from build123d import *

# Parameters (mm, degrees)
SKETCH1_W           = 25
SKETCH1_H           = 23.86
BOSS_EXTRUDE1_DEPTH = 1.12
SKETCH4_W           = 10.8
SKETCH4_H           = 10.8
BOSS_EXTRUDE2_DEPTH = 3.875
SKETCH5_R           = 2.375
CUT_EXTRUDE1_DEPTH  = 0.7
CUT_EXTRUDE2_REACH  = 19.708
SKETCH6_R           = 1.1
SKETCH8_R           = 1
BOSS_EXTRUDE3_DEPTH = 6.98
SKETCH9_W           = 25
SKETCH9_H           = 5.71
BOSS_EXTRUDE4_DEPTH = 2.75
FILLET1_R           = 1.5


with BuildPart() as part:
    # Sketch1 → Boss-Extrude1 (new body)
    with BuildSketch(Plane.XY):
        Rectangle(SKETCH1_W, SKETCH1_H)
    extrude(amount=BOSS_EXTRUDE1_DEPTH)

    # Sketch4 → Boss-Extrude2 (add)
    with BuildSketch(Plane.XY.offset(1.12)):
        with Locations((0, 2.2016)):
            Rectangle(SKETCH4_W, SKETCH4_H)
    extrude(amount=BOSS_EXTRUDE2_DEPTH)

    # Sketch5 → Cut-Extrude1 (cut)
    with BuildSketch(Plane.XY.offset(1.12)):
        with Locations((11, 2.2016)):
            Circle(SKETCH5_R)
        with Locations((11, -10.4984)):
            Circle(SKETCH5_R)
        with Locations((-11, -10.4984)):
            Circle(SKETCH5_R)
        with Locations((-11, 2.2016)):
            Circle(SKETCH5_R)
    extrude(amount=-CUT_EXTRUDE1_DEPTH, mode=Mode.SUBTRACT)

    # Sketch6 → Cut-Extrude2 (cut, up to next)
    with BuildSketch(Plane.XY.offset(1.12), mode=Mode.PRIVATE) as cut_extrude2_sk1:
        with Locations((11, 2.2016)):
            Circle(SKETCH6_R)
    cut_extrude2_tool1 = extrude(cut_extrude2_sk1.sketch, amount=-CUT_EXTRUDE2_REACH, mode=Mode.PRIVATE) & part.part
    # Sketch6 → Cut-Extrude2 (cut, up to next)
    with BuildSketch(Plane.XY.offset(1.12), mode=Mode.PRIVATE) as cut_extrude2_sk2:
        with Locations((11, -10.4984)):
            Circle(SKETCH6_R)
    cut_extrude2_tool2 = extrude(cut_extrude2_sk2.sketch, amount=-CUT_EXTRUDE2_REACH, mode=Mode.PRIVATE) & part.part
    # Sketch6 → Cut-Extrude2 (cut, up to next)
    with BuildSketch(Plane.XY.offset(1.12), mode=Mode.PRIVATE) as cut_extrude2_sk3:
        with Locations((-11, -10.4984)):
            Circle(SKETCH6_R)
    cut_extrude2_tool3 = extrude(cut_extrude2_sk3.sketch, amount=-CUT_EXTRUDE2_REACH, mode=Mode.PRIVATE) & part.part
    # Sketch6 → Cut-Extrude2 (cut, up to next)
    with BuildSketch(Plane.XY.offset(1.12), mode=Mode.PRIVATE) as cut_extrude2_sk4:
        with Locations((-11, 2.2016)):
            Circle(SKETCH6_R)
    cut_extrude2_tool4 = extrude(cut_extrude2_sk4.sketch, amount=-CUT_EXTRUDE2_REACH, mode=Mode.PRIVATE) & part.part
    add(cut_extrude2_tool1.solids().sort_by_distance((11, 2.2016, 1.12))[0], mode=Mode.SUBTRACT)
    add(cut_extrude2_tool2.solids().sort_by_distance((11, -10.4984, 1.12))[0], mode=Mode.SUBTRACT)
    add(cut_extrude2_tool3.solids().sort_by_distance((-11, -10.4984, 1.12))[0], mode=Mode.SUBTRACT)
    add(cut_extrude2_tool4.solids().sort_by_distance((-11, 2.2016, 1.12))[0], mode=Mode.SUBTRACT)

    # Sketch8 → Boss-Extrude3 (add)
    with BuildSketch(Plane.XY.offset(1.12)):
        with BuildLine():
            Line((2.875, 4.0766), (2.875, 0.3266))
            ThreePointArc((2.875, 0.3266), (2.582106781, -0.380506781), (1.875, -0.6734))
            Line((1.875, -0.6734), (-1.875, -0.6734))
            ThreePointArc((-1.875, -0.6734), (-2.582106781, -0.380506781), (-2.875, 0.3266))
            Line((-2.875, 0.3266), (-2.875, 4.0766))
            ThreePointArc((-2.875, 4.0766), (-2.582106781, 4.783706781), (-1.875, 5.0766))
            Line((-1.875, 5.0766), (1.875, 5.0766))
            ThreePointArc((1.875, 5.0766), (2.582106781, 4.783706781), (2.875, 4.0766))
        make_face()
        with Locations((0, 2.2016)):
            Circle(SKETCH8_R, mode=Mode.SUBTRACT)
    extrude(amount=BOSS_EXTRUDE3_DEPTH)

    # Sketch9 → Boss-Extrude4 (add)
    with BuildSketch(Plane(origin=(0, 0, 0), x_dir=(-1, 0, 0), z_dir=(0, 0, -1))):
        with Locations((0, 9.075)):
            Rectangle(SKETCH9_W, SKETCH9_H)
    extrude(amount=BOSS_EXTRUDE4_DEPTH)

    # Fillet1
    fillet1_edges = [part.edges().sort_by_distance(p)[0] for p in [
        (12.5, -11.93, 0.21),
        (-12.5, -11.93, 0.21),
        (12.5, 11.93, -0.815),
        (-12.5, 11.93, -0.815),
    ]]
    fillet(fillet1_edges, radius=FILLET1_R)


solid = part.part
Here's how the part is built. I have some questions about the finished solid (model axes, mm). A direction names the side the tool comes from. Give positions to 0.01 mm unless a question says otherwise; leave off trailing zeros. Write each loop counter-clockwise with the first axis right and the second up, starting at its lowest first coordinate (ties: lowest second). Pieces come first, ordered by that corner, then holes. Notation, with made-up numbers: (42.25, -12.75) -> (89.25, -12.75) arc R34 cw to (89.25, 18.25) -> close; hole circle Ø6 at (34, 43). An arc over 180 degrees is marked (long way). Use one line per item in the form item = value. Start each with the question number.
1. If I drill on L1, parallel to Y at x = 11, z = 0.3; L2, parallel to Z at x = 1.5, y = -9; L3, parallel to Z at x = 11, y = 7.5, over which ranges is the centre line in solid material (lowest first)?
2. Imagine slicing it at C-C on z = -0.5. List the corners of the cut face in (x, y) for me.
3. Imagine slicing it at B-B on y = 7. List the corners of the cut face in (x, z) for me (3 decimals).
4. Imagine slicing it at D-D on x = 10.5. List the corners of the cut face in (y, z) for me.
5. Will these pins go through, and if not, where does the flat tip stop? pin 1 Ø3 at (x, y) = (-10.5, -10) entering from +Z; pin 2 Ø3.5 at (x, y) = (11, -10.5) entering from -Z; pin 3 Ø2.5 at (x, z) = (0, 6.5) entering from -Y; pin 4 Ø1.5 at (x, z) = (-10, 2.5) entering from -Y.
6. Thinking about a two-plate mould opening in Y: for faces 5 (the face through (-12.07, 11.48, -0.79)), 6 (the face through (-9.32, -8.82, 0.77)), 7 (the face through (-2.57, -0.39, 6.53)), which applies, +Y half, -Y half, draft (parallel to the pull), parting line (faces both ways), or undercut?
7. On a 3-axis mill with a long thin cutter (end or side, diameter ignored), from which of +Z, -Z, +X, -X, +Y, -Y can I reach the whole of each face in a straight line? I mean faces 1 (the face through (-9.7, 2.2, 0.42)), 2 (the face through (0, -3, 0)), 3 (the face through (0, -3.198, 3)), 4 (the face through (-2.875, 2, 7)). Say none if no direction works.
8. Imagine slicing it at A-A on x = -1.5. List the corners of the cut face in (y, z) for me (3 decimals), plus the area to 3 significant figures.
Entries:
q1.L1 = -11.93 to -11.6, -9.4 to 1.1, 3.3 to 11.93
q1.L2 = 0 to 1.12
q1.L3 = -2.75 to 1.12
q2.outline = (-12.5, 6.22) -> (12.5, 6.22) -> (12.5, 10.43) arc R1.5 ccw to (11, 11.93) -> (-11, 11.93) arc R1.5 ccw to (-12.5, 10.43) -> close
q3.outline = (-12.5, -2.75) -> (12.5, -2.75) -> (12.5, 1.12) -> (5.4, 1.12) -> (5.4, 4.995) -> (-5.4, 4.995) -> (-5.4, 1.12) -> (-12.5, 1.12) -> close
q4.outline = (-11.93, 0) -> (-11.48, 0) -> (-11.48, 0.42) -> (-11.93, 0.42) -> close; (-9.52, 0) -> (1.22, 0) -> (1.22, 0.42) -> (-0.12, 0.42) -> (-0.12, 1.12) -> (-8.18, 1.12) -> (-8.18, 0.42) -> (-9.52, 0.42) -> close; (3.18, 0) -> (6.22, 0) -> (6.22, -2.75) -> (11.93, -2.75) -> (11.93, 1.12) -> (4.52, 1.12) -> (4.52, 0.42) -> (3.18, 0.42) -> close
q5.pin_1 = 0.42
q5.pin_2 = 0
q5.pin_3 = -0.67
q5.pin_4 = through
q6.face_5 = +Y half
q6.face_6 = undercut
q6.face_7 = -Y half
q7.face_1 = +Z
q7.face_2 = -Z, +X, -X, -Y
q7.face_3 = +Z, +X, -X, -Y
q7.face_4 = +Z, -X, +Y, -Y
q8.outline = (-11.93, 0) -> (6.22, 0) -> (6.22, -2.75) -> (11.93, -2.75) -> (11.93, 1.12) -> (7.602, 1.12) -> (7.602, 4.995) -> (5.077, 4.995) -> (5.077, 8.1) -> (-0.673, 8.1) -> (-0.673, 4.995) -> (-3.198, 4.995) -> (-3.198, 1.12) -> (-11.93, 1.12) -> close
q8.area = 102 mm²
